Here's the drawing with two shaded views (mm, measured from the low corner). I have some questions. Coordinates: 2 decimals unless noted, no trailing zeros. Loops run counter-clockwise (first coordinate to the right, second up) from the corner with the lowest first, then second, coordinate; pieces in that order, holes last. Notation, with made-up numbers: M 61,73 L 94,73 A27 ccw 94,99 Z; hole C -6,56 d10. An arc over 180 degrees is marked long. Return JSON: item names as keys, results as strings. Group by question number.
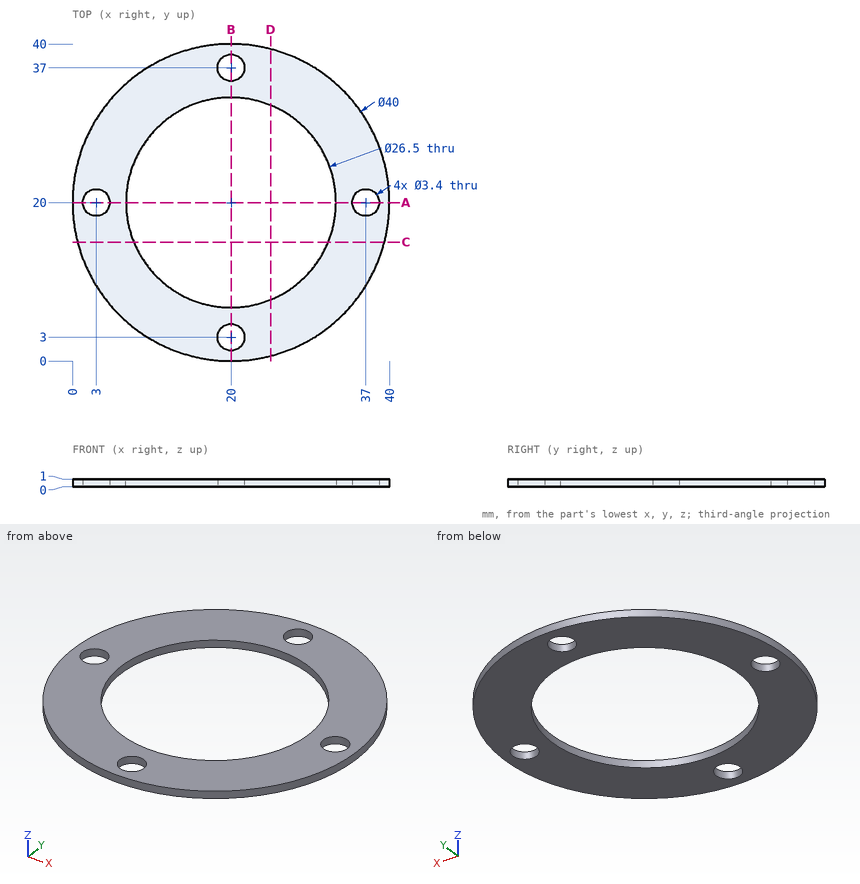
(1) Will this pin go through, and if not, where does the flat tip stop? P1, Ø2.5, axis at x = 37, y = 20, coming from the +Z side.
(2) Imagine slicing it at C-C, the plane y = 15. Write out the boundary of the cut face in (x, z), then the cut area to 3 significant figures.
(3) Imagine slicing it at A-A, the plane y = 20. Write out the boundary of the cut face in (x, z), then the cut area to 3 significant figures.
(4) If I drill on L1, parallel to X at y = 19, z = 0.3; L2, parallel to X at y = 18, z = 0.35, over which ranges is the centre line in solid material (lowest first)? Write a range as [from, to].
Checks:
{
 "1": {"P1": "through"},
 "2": {"outline": "M 0.64,0 L 7.73,0 L 7.73,1 L 0.64,1 Z; M 32.27,0 L 39.36,0 L 39.36,1 L 32.27,1 Z", "area": "14.2 mm²"},
 "3": {"outline": "M 0,0 L 1.3,0 L 1.3,1 L 0,1 Z; M 4.7,0 L 6.75,0 L 6.75,1 L 4.7,1 Z; M 33.25,0 L 35.3,0 L 35.3,1 L 33.25,1 Z; M 38.7,0 L 40,0 L 40,1 L 38.7,1 Z", "area": "6.70 mm²"},
 "4": {"L1": "[0.03, 1.63], [4.37, 6.79], [33.21, 35.63], [38.37, 39.97]", "L2": "[0.1, 6.9], [33.1, 39.9]"}
}
